Verification items for the finished model (mm, model axes). A direction names the side the tool comes from. Give positions to 0.01 mm unless a question says otherwise; leave off trailing zeros. Order: outer loops, then holes, each group sorted by start corner. A loop starts at its lowest first (then second) coordinate and runs counter-clockwise, first axis right, second up. Notation, with made-up numbers: M 84,86 L 110,86 A31 cw 110,123 Z; hole C 62.5,1 d1. An arc over 180 degrees is marked long. Answer as a JSON object with one key per item and string values.
Autodesk Inventor part; units mm, degrees
ref_plane "YZ Plane" through (0, 0, 0) normal (1, 0, 0) x (0, 1, 0)
ref_plane "XZ Plane" through (0, 0, 0) normal (0, 1, 0) x (-1, 0, 0)
ref_plane "XY Plane" through (0, 0, 0) normal (0, 0, 1) x (1, 0, 0)
sketch "Sketch1" plane through (0, 0, 0) normal (1, 0, 0) x (0, 1, 0)
  line L0 (0, 0) -> (15, 0)
  line L1 (15, 0) -> (15, -30)
  line L2 (15, -30) -> (0, -30)
  line L3 (0, -30) -> (0, 0)
  line L4 (0, -8.4131) -> (10, -3.75)
  line L5 (10, -3.75) -> (10, -26.25)
  line L6 (10, -26.25) -> (0, -21.5869)
  point P0 (10, -15)
  point P1 (0, -15)
  dimension "d0" = 15
  dimension "d1" = 30
  dimension "d2" = 10
  dimension "d3" = 22.5
  dimension "d4" = 65
  dimension "d5" = 65
extrude "Extrusion1" add sketch "Sketch1" along normal blind 30 contours L0 L1 L2 L3 L6 L5 L4
sketch "Sketch2" plane through (30, 0, 0) normal (1, 0, 0) x (0, 0, -1)
  line L0 (0, 15) -> (0, 0)
  line L1 (21.5869, 0) -> (30, 0)
  line L2 (0, 15) -> (30, 15)
  line L3 (30, 15) -> (30, 0)
  line L4 (30, 0) -> (0, 0)
  line L5 (0, 0) -> (0, 15)
extrude "Extrusion2" add sketch "Sketch2" along normal blind 2.5
sketch "Sketch3" plane through (0, 0, 0) normal (-1, 0, 0) x (0, 0, 1)
  line L0 (-30, 0) -> (-30, 15)
  line L1 (0, 15) -> (0, 0)
  line L2 (-30, 15) -> (0, 15)
  line L3 (0, 15) -> (0, 10)
  line L4 (0, 10) -> (-30, 10)
  line L5 (-30, 10) -> (-30, 15)
  dimension "d10" = 5
extrude "Extrusion3" add sketch "Sketch3" along normal blind 5
sketch "Sketch4" plane through (32.5, 15, 0) normal (0, 1, 0) x (1, 0, 0)
  line L0 (-32.5, 0) -> (-37.5, 0)
  line L1 (-32.5, 0) -> (-32.5, 30) construction
  circle A0 centre (-35, 15) radius 1.5
  dimension "d13" = 3
extrude "Extrusion4" cut sketch "Sketch4" against normal through all
properties part number "Top Sensor Mount"
Q1. Gauge pin test, flat ends, axial feed: pin 1 Ø6.5 at (y, z) = (3, -6) entering from -X; pin 2 Ø3.5 at (x, z) = (-2.5, -15) entering from -Y; pin 3 Ø5 at (x, z) = (9, -4) entering from -Y; pin 4 Ø3 at (y, z) = (3, -12) entering from -X. Record the tip position at first contact, or that the pin passes through.
Resolved:
{"pin 1": "stops at x = 0", "pin 2": "stops at y = 10", "pin 3": "stops at y = 0", "pin 4": "stops at x = 30"}
Q2. Release check for a two-part mould opening along Y. For faces 4 (the face through (14, 15, -15)), 5 (the face through (0, 4, -27)), 6 (the face through (13, 10, -15)), 7 (the face through (14.79, 4.93, -6.114)) record: +Y half, -Y half, draft (parallel to the pull), parting line (faces both ways), or undercut.
Resolved:
{"face 4": "+Y half", "face 5": "draft", "face 6": "undercut", "face 7": "undercut"}
Q3. Section check D-D on y = 2.25. Record the cut outline in (x, z), then the cut area to 3 significant figures.
Resolved:
{"outline": "M 0,-30 L 32.5,-30 L 32.5,0 L 0,0 L 0,-7.36 L 30,-7.36 L 30,-22.64 L 0,-22.64 Z", "area": "517 mm²"}
Q4. Section check A-A on z = -15. Record the cut outline in (x, y).
Resolved:
{"outline": "M -5,10 L -4,10 L -4,15 L -5,15 Z; M -1,10 L 30,10 L 30,0 L 32.5,0 L 32.5,15 L -1,15 Z"}
Q5. Section check C-C on x = 22. Record the cut outline in (y, z).
Resolved:
{"outline": "M 0,-30 L 15,-30 L 15,0 L 0,0 L 0,-8.41 L 10,-3.75 L 10,-26.25 L 0,-21.59 Z"}
Q6. Section check B-B on x = -2.5. Record the cut outline in (y, z).
Resolved:
{"outline": "M 10,-30 L 15,-30 L 15,-16.5 L 10,-16.5 Z; M 10,-13.5 L 15,-13.5 L 15,0 L 10,0 Z"}
Q7. Material ranges on L1, parallel to X at y = 11.6, z = -15; L2, parallel to Z at x = -2.5, y = 13.95; L3, parallel to Y at x = 29.5, z = -19.5, recorded low to high.
Resolved:
{"L1": "x = -5 to -4, -1 to 32.5", "L2": "z = -30 to -16.5, -13.5 to 0", "L3": "y = 10 to 15"}
Q8. Tool access check on faces 1 (the face through (14.79, 5.07, -23.95)), 2 (the face through (0, 4, -3)), 3 (the face through (14, 8, 0)). Record the directions out of +Z, -Z, +X, -X, +Y, -Y that give a thin tool (end or side, any length) a straight path to the whole face; none if there is none.
Resolved:
{"face 1": "-X", "face 2": "+Z, -Z, -X, -Y", "face 3": "+Z, +X, -X, +Y, -Y"}
